Job drawing, mm, ordinate dimensions from the low corner. One solid piece. A direction names the side the tool comes from. Give positions to 0.01 mm unless a question says otherwise; leave off trailing zeros. Order: outer loops, then holes, each group sorted by start corner. A loop starts at its lowest first (then second) coordinate and runs counter-clockwise, first axis right, second up. Notation, with made-up numbers: (58, 16.25) -> (117, 16.25) arc R13 cw to (117, 32.25) -> close; hole circle Ø3 at (14.5, 84.5). An arc over 180 degrees is marked (long way). Write item = value, one per line. Start each with the question number.
(1) Two-plate mould, pull along X, no slides. Class the marked faces 1, 2 and 3: pulls with the +X half, pulls with the -X half, needs draft (parallel to the pull), parting line crosses it, or undercut.
(2) Flat gauge pins, fed straight in: pin 1 (3 mm diameter, centred on x = 32, z = 19.5, fed in from -Y); pin 2 (1 mm diameter, centred on y = 3.5, z = 11, fed in from -X); pin 3 (2.5 mm diameter, centred on x = 24.5, z = 3.25, fed in from +Y); pin 4 (2 mm diameter, centred on y = 5, z = 39.5, fed in from +X). Where does each tip first touch, or does it go through?
(3) Saw through at B-B, the plane z = 45.75. List the corners of the cut face in (x, y), then the cut area to 3 significant figures.
(4) Saw through at C-C, the plane x = 10.5. List the corners of the cut face in (y, z).
(5) Saw through at D-D, the plane z = 24.5. List the corners of the cut face in (x, y), then the cut area to 3 significant figures.
(6) Probe line 1 along X through (y, z) = (1.45, 24.5); line 2 along Y through (x, z) = (40.5, 20); line 3 along X through (y, z) = (2.25, 3.25). List the from-to ranges inside material, lowest first. Write a range as from..to.
(7) Which spindle directions (+Z, -Z, +X, -X, +Y, -Y) get a long thin tool onto all of the face, cutting with end or side? Do the marked faces 4 and 5. Say none if no direction does.
(8) Saw through at A-A, the plane y = 2.75. List the corners of the cut face in (x, z).
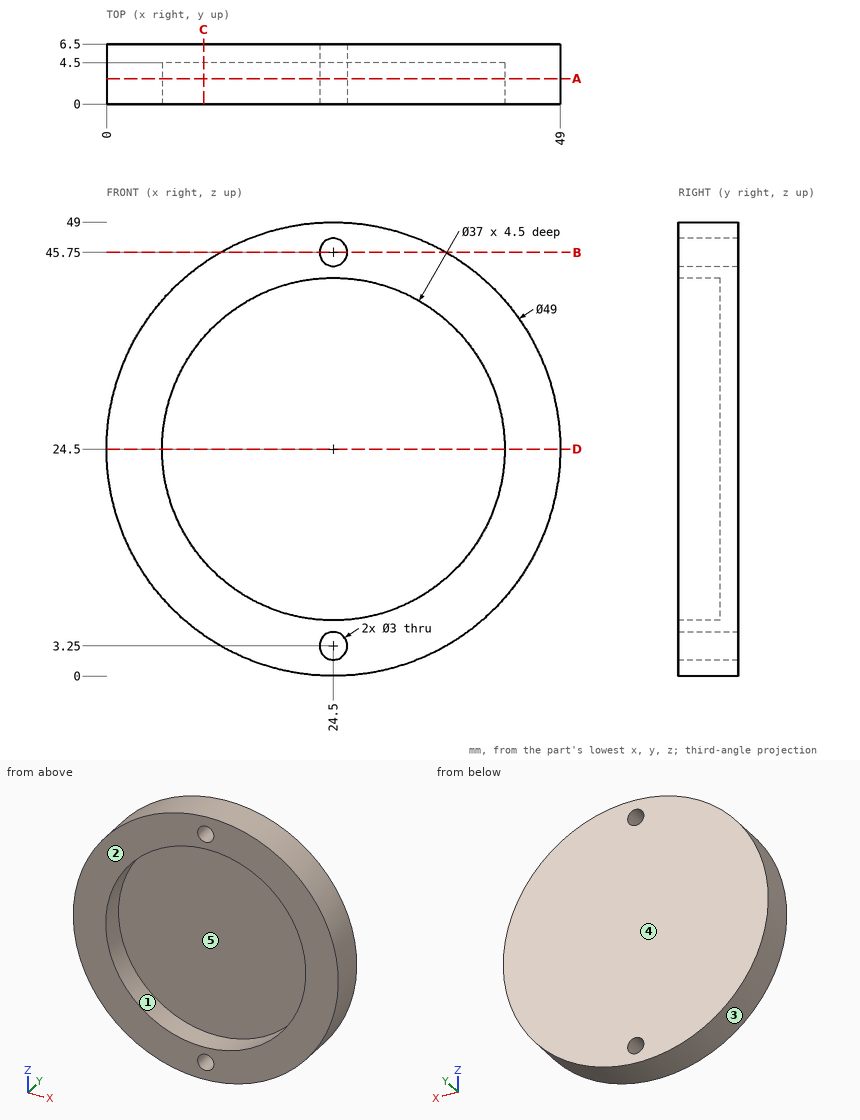
Results list:
q1.face_1 = undercut
q1.face_2 = needs draft
q1.face_3 = parting line crosses it
q2.pin_1 = 4.5
q2.pin_2 = 3.73
q2.pin_3 = through
q2.pin_4 = 44.61
q3.outline = (12.31, 0) -> (23, 0) -> (23, 6.5) -> (12.31, 6.5) -> close; (26, 0) -> (36.69, 0) -> (36.69, 6.5) -> (26, 6.5) -> close
q3.area = 139 mm^2
q4.outline = (0, 4.39) -> (6.5, 4.39) -> (6.5, 44.61) -> (0, 44.61) -> (0, 36.59) -> (4.5, 36.59) -> (4.5, 12.41) -> (0, 12.41) -> close
q5.outline = (0, 0) -> (6, 0) -> (6, 4.5) -> (43, 4.5) -> (43, 0) -> (49, 0) -> (49, 6.5) -> (0, 6.5) -> close
q5.area = 152 mm^2
q6.line_1 = 0..6, 43..49
q6.line_2 = 4.5..6.5
q6.line_3 = 12.31..23, 26..36.69
q7.face_4 = +Z, -Z, +X, -X, +Y
q7.face_5 = -Y
q8.outline = circle Ø49 at (24.5, 24.5); hole circle Ø37 at (24.5, 24.5); hole circle Ø3 at (24.5, 3.25); hole circle Ø3 at (24.5, 45.75)
